Verification items for this drawing (mm, ordinates from the low corner). A direction names the side the tool comes from. Round coordinates to 2 decimals unless told otherwise and drop trailing zeros. Write each loop counter-clockwise with the first axis right and the second up, starting at its lowest first coordinate (ties: lowest second). Pieces come first, ordered by that corner, then holes. Notation, with made-up numbers: M 25.5,75.25 L 61.5,75.25 A24 cw 61.5,110.25 Z; hole C 72,-21.75 d6. An arc over 180 degrees is marked long. Write each question's results on one line, items separated by ' | '.
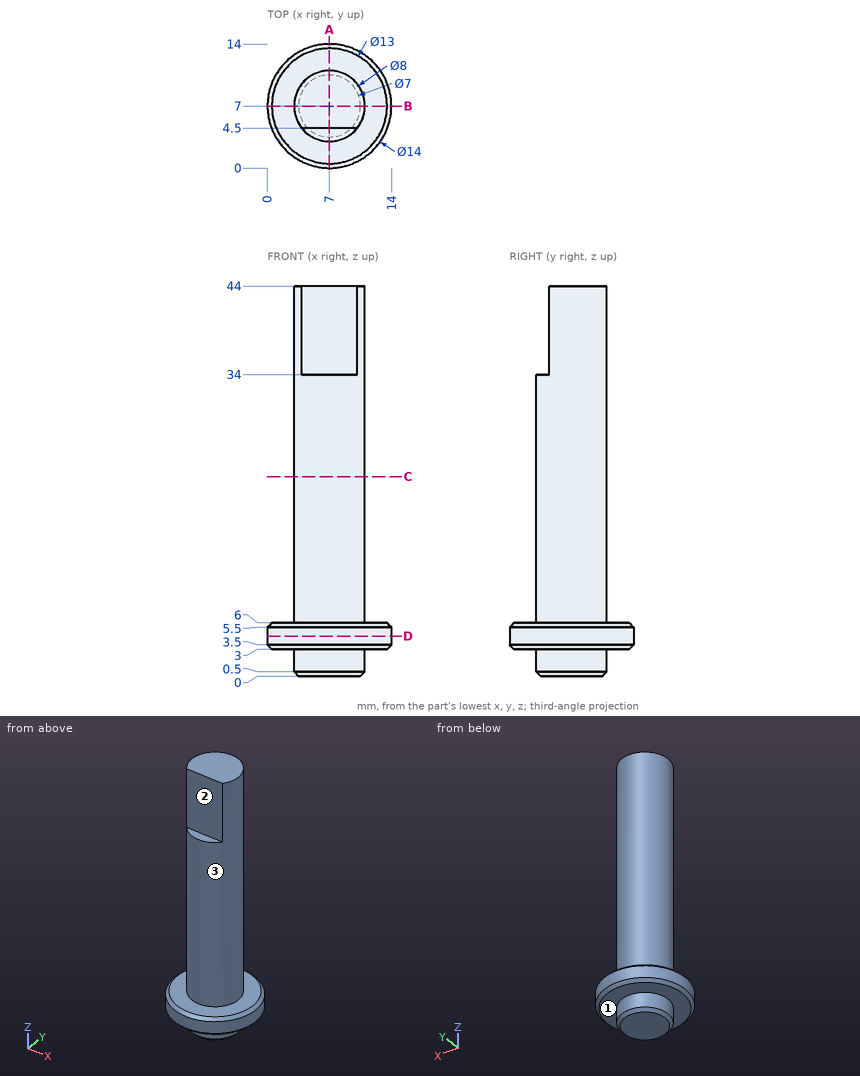
1) Depth check by flat-ended pin: P1, Ø1, axis at x = 4.5, z = 27, coming from the -Y side; P2, Ø2, axis at x = 12.5, y = 11.5, coming from the -Z side; P3, Ø4, axis at x = 6, z = 29.5, coming from the +Y side. Enter the tip coordinate at first touch or a pass-through.
Calculated:
P1: stops at y = 3.54 | P2: stops at z = 3 | P3: stops at y = 11
2) Material ranges on line 1 (X direction, y = 4.5, z = 29); line 2 (Z direction, x = 9.5, y = 1.25); line 3 (X direction, y = 10.5, z = 29), recorded low to high. Write a range as [from, to].
Calculated:
line 1: x = [3.88, 10.12] | line 2: z = [3, 6] | line 3: x = [5.06, 8.94]
3) Sectioned sample at A-A, the plane x = 7. Record the cut outline in (y, z).
Calculated:
outline: M 0,3.5 L 0.5,3 L 3,3 L 3,0.5 L 3.5,0 L 10.5,0 L 11,0.5 L 11,3 L 13.5,3 L 14,3.5 L 14,5.5 L 13.5,6 L 11,6 L 11,44 L 4.5,44 L 4.5,34 L 3,34 L 3,6 L 0.5,6 L 0,5.5 Z
4) Access from +Z, -Z, +X, -X, +Y, -Y to the whole of each face (thin tool, end or side, straight path). Record for the marked faces 1, 2 and 3.
Calculated:
face 1: -Z | face 2: +Z, +X, -X, -Y | face 3: +Z
5) Sectioned sample at C-C, the plane z = 22.5. Record the cut outline in (x, y), and give its area (3 significant figures).
Calculated:
outline: C 7,7 d8 | area: 50.3 mm²
6) Sectioned sample at B-B, the plane y = 7. Record the cut outline in (x, z).
Calculated:
outline: M 0,3.5 L 0.5,3 L 3,3 L 3,0.5 L 3.5,0 L 10.5,0 L 11,0.5 L 11,3 L 13.5,3 L 14,3.5 L 14,5.5 L 13.5,6 L 11,6 L 11,44 L 3,44 L 3,6 L 0.5,6 L 0,5.5 Z
7) Sectioned sample at D-D, the plane z = 4.5. Record the cut outline in (x, y).
Calculated:
outline: C 7,7 d14
